```python
from build123d import *

# Parameters (mm, degrees)
SKETCH_2_W          = 129
SKETCH_2_H          = 73
EXTRUDE_1_DEPTH     = 1.5
SKETCH_2_4_W        = 2
SKETCH_2_4_H        = 69
EXTRUDE_2_DEPTH     = 30
SKETCH_2_5_W        = 129
SKETCH_2_5_H        = 2
EXTRUDE_3_DEPTH     = 30
SKETCH_2_6_W        = 129
SKETCH_2_6_H        = 2
EXTRUDE_4_DEPTH     = 30
SKETCH_5_W          = 45
SKETCH_5_H          = 2
CUT_EXTRUDE_2_DEPTH = 14
SKETCH_6_W          = 20
SKETCH_6_H          = 2
CUT_EXTRUDE_3_DEPTH = 14
FILLET_1_R          = 1
FILLET_2_R          = 1
FILLET_5_R          = 1
SKETCH_8_R          = 3.5
CUT_EXTRUDE_4_DEPTH = 10
FILLET_6_R          = 1
EXTRUDE_5_DEPTH     = 30


with BuildPart() as part:
    # 草图2 → 凸台-拉伸1 (new body)
    with BuildSketch(Plane(origin=(0, 0, 0), x_dir=(1, 0, 0), z_dir=(0, 1, 0))):
        Rectangle(SKETCH_2_W, SKETCH_2_H)
    extrude(amount=EXTRUDE_1_DEPTH)

    # 草图2<4> → 凸台-拉伸2 (add)
    with BuildSketch(Plane(origin=(0, 0, 0), x_dir=(1, 0, 0), z_dir=(0, 1, 0))):
        with Locations((-63.5, 0)):
            Rectangle(SKETCH_2_4_W, SKETCH_2_4_H)
    extrude(amount=-EXTRUDE_2_DEPTH)

    # 草图2<5> → 凸台-拉伸3 (add)
    with BuildSketch(Plane(origin=(0, 0, 0), x_dir=(1, 0, 0), z_dir=(0, 1, 0))):
        with Locations((0, 35.5)):
            Rectangle(SKETCH_2_5_W, SKETCH_2_5_H)
    extrude(amount=-EXTRUDE_3_DEPTH)

    # 草图2<6> → 凸台-拉伸4 (add)
    with BuildSketch(Plane(origin=(0, 0, 0), x_dir=(1, 0, 0), z_dir=(0, 1, 0))):
        with Locations((0, -35.5)):
            Rectangle(SKETCH_2_6_W, SKETCH_2_6_H)
    extrude(amount=-EXTRUDE_4_DEPTH)

    # 草图5 → 切除-拉伸2 (cut)
    with BuildSketch(Plane.XZ.offset(30)):
        with Locations((35, 35.5)):
            Rectangle(SKETCH_5_W, SKETCH_5_H)
    extrude(amount=-CUT_EXTRUDE_2_DEPTH, mode=Mode.SUBTRACT)

    # 草图6 → 切除-拉伸3 (cut)
    with BuildSketch(Plane.XZ.offset(30)):
        with Locations((37.5, -35.5)):
            Rectangle(SKETCH_6_W, SKETCH_6_H)
    extrude(amount=-CUT_EXTRUDE_3_DEPTH, mode=Mode.SUBTRACT)

    # 圆角1
    fillet_1_edges = [part.edges().sort_by_distance(p)[0] for p in [
        (-64.5, -14.25, -36.5),
    ]]
    fillet(fillet_1_edges, radius=FILLET_1_R)

    # 圆角2
    fillet_2_edges = [part.edges().sort_by_distance(p)[0] for p in [
        (-64.5, -14.25, 36.5),
    ]]
    fillet(fillet_2_edges, radius=FILLET_2_R)

    # 圆角5
    fillet_5_edges = [part.edges().sort_by_distance(p)[0] for p in [
        (64.5, -14.25, 36.5),
    ]]
    fillet(fillet_5_edges, radius=FILLET_5_R)

    # 草图8 → 切除-拉伸4 (cut)
    with BuildSketch(Plane(origin=(0, 1.5, 0), x_dir=(1, 0, 0), z_dir=(0, 1, 0))):
        with Locations((-34.5, 30.7)):
            Circle(SKETCH_8_R)
        with Locations((56.5, 30.7)):
            Circle(SKETCH_8_R)
        with Locations((-34.5, -30.7)):
            Circle(SKETCH_8_R)
        with Locations((56.5, -30.7)):
            Circle(SKETCH_8_R)
    extrude(amount=-CUT_EXTRUDE_4_DEPTH, mode=Mode.SUBTRACT)

    # 圆角6
    fillet_6_edges = [part.edges().sort_by_distance(p)[0] for p in [
        (64.5, -14.25, -36.5),
    ]]
    fillet(fillet_6_edges, radius=FILLET_6_R)

    # 草图9 → 凸台-拉伸5 (add)
    with BuildSketch(Plane.XZ):
        Polygon((62.5, 34.5), (64.5, 34.5), (64.5, 32.5), (63.5, 32.5), (63.5, 31.5), (62.5, 31.5), align=None)
        Polygon((62.5, -34.5), (62.5, -31.5), (63.5, -31.5), (63.5, -32.5), (64.5, -32.5), (64.5, -34.5), align=None)
    extrude(amount=EXTRUDE_5_DEPTH)


solid = part.part
```
For this review, take the finished solid that the model builds, in its own axes (mm). A direction names the side the tool comes from. Round coordinates to 2 decimals unless told otherwise and drop trailing zeros. Order: outer loops, then holes, each group sorted by start corner. A loop starts at its lowest first (then second) coordinate and runs counter-clockwise, first axis right, second up.
Q1. We need section B-B, the plane y = -26. Give the boundary of the cut face in (x, z), plus the area to 3 significant figures.
Findings below:
outline: (-64.5, -35.5) arc R1 ccw to (-63.5, -36.5) - (27.5, -36.5) - (27.5, -34.5) - (-62.5, -34.5) - (-62.5, 34.5) - (12.5, 34.5) - (12.5, 36.5) - (-63.5, 36.5) arc R1 ccw to (-64.5, 35.5) - close; (47.5, -36.5) - (63.5, -36.5) arc R1 ccw to (64.5, -35.5) - (64.5, -32.5) - (63.5, -32.5) - (63.5, -31.5) - (62.5, -31.5) - (62.5, -34.5) - (47.5, -34.5) - close; (57.5, 34.5) - (62.5, 34.5) - (62.5, 31.5) - (63.5, 31.5) - (63.5, 32.5) - (64.5, 32.5) - (64.5, 35.5) arc R1 ccw to (63.5, 36.5) - (57.5, 36.5) - close
area: 533 mm2
Q2. Machinability: for faces 5 (the flat face through (62.5, -15, 33)), 6 (the flat face through (-15, -11, 36.5)), which of the approach directions +Z, -Z, +X, -X, +Y, -Y give a long, thin tool a straight path to every point of the face, cutting with its end or side? Answer none if there is none.
Findings below:
face 5: -Y
face 6: +Z, +X, -X, +Y, -Y
Q3. We need section C-C, the plane y = -4.5. Give the boundary of the cut face in (x, z).
Findings below:
outline: (-64.5, -35.5) arc R1 ccw to (-63.5, -36.5) - (63.5, -36.5) arc R1 ccw to (64.5, -35.5) - (64.5, -32.5) - (63.5, -32.5) - (63.5, -31.5) - (62.5, -31.5) - (62.5, -34.5) - (-62.5, -34.5) - (-62.5, 34.5) - (62.5, 34.5) - (62.5, 31.5) - (63.5, 31.5) - (63.5, 32.5) - (64.5, 32.5) - (64.5, 35.5) arc R1 ccw to (63.5, 36.5) - (-63.5, 36.5) arc R1 ccw to (-64.5, 35.5) - close
Q4. We need section A-A, the plane x = -34.5. Give the boundary of the cut face in (y, z).
Findings below:
outline: (-30, -36.5) - (1.5, -36.5) - (1.5, -34.2) - (0, -34.2) - (0, -34.5) - (-30, -34.5) - close; (-30, 34.5) - (0, 34.5) - (0, 34.2) - (1.5, 34.2) - (1.5, 36.5) - (-30, 36.5) - close; (0, -27.2) - (1.5, -27.2) - (1.5, 27.2) - (0, 27.2) - close
Q5. We need section D-D, the plane x = 19. Give the boundary of the cut face in (y, z), plus the area to 4 significant figures.
Findings below:
outline: (-30, -36.5) - (1.5, -36.5) - (1.5, 36.5) - (-16, 36.5) - (-16, 34.5) - (0, 34.5) - (0, -34.5) - (-30, -34.5) - close
area: 201.5 mm2
Q6. Mouldability with a two-part tool opening along X and no side actions: class faces 1 (the cylindrical face through (53.003, 0.76, 30.546)), 2 (the flat face through (-64.5, -14, 0)), 3 (the flat face through (-1, -15, -34.5)), 4 (the flat face through (-63, -30, -3)) as pulls with the +X half, pulls with the -X half, needs draft (parallel to the pull), parting line crosses it, or undercut.
Findings below:
face 1: undercut
face 2: pulls with the -X half
face 3: undercut
face 4: needs draft
Q7. Insertion check: P1, Ø5, axis at y = -9, z = 27, coming from the +X side; P2, Ø9, axis at x = 56.5, z = -30.7, coming from the +Y side; P3, Ø4, axis at x = -9, z = -22.5, coming from the -Y side; P4, Ø1, axis at x = 37, z = -35, coming from the -Y side. Each pin has a flat end and moves straight along its axis. Give the tip position at first contact, or say it passes through.
Findings below:
P1: stops at x = -62.5
P2: stops at y = 1.5
P3: stops at y = 0
P4: stops at y = -16
Q8. Wall thickness on line 1 (Z direction, x = -34.5, y = 1.2); line 2 (X direction, y = 0.6, z = 30.7); line 3 (Z direction, x = -53, y = -16.5): over which ranges is each line inside the solid? List them lowest first.
Findings below:
line 1: z = -36.5 to -34.2, -27.2 to 27.2, 34.2 to 36.5
line 2: x = -64.5 to -38, -31 to 53, 60 to 64.5
line 3: z = -36.5 to -34.5, 34.5 to 36.5
